Source: CAD feature listing. Evaluate the final solid. Frame: model axes, mm. Face numbers are marked on the shaded views. A direction names the side the tool comes from. Coordinates: 2 decimals unless noted, no trailing zeros. Order: outer loops, then holes, each group sorted by start corner. A loop starts at its lowest first (then second) coordinate and runs counter-clockwise, first axis right, second up.
Item 1: Section C-C on x = 0. Return the cut outline in (y, z) (3 decimals), then the cut area to 3 significant figures.
Item 2: Ray query, line 1 (X direction, y = 42, z = -19.05); line 2 (X direction, y = 58.5, z = -17); line 3 (Z direction, x = 3, y = 45). Return the intervals inside material, ascending.
Item 3: Section D-D on z = 3. Return the cut outline in (x, y), then the cut area to 3 significant figures.
Item 4: Mould query, pull axis Y, two halves, no side actions, for the marked faces 5, 6, 7 and 8. Classes: released by +Y, released by -Y, zero draft, split by the parting line, or undercut.
Item 5: Contact query for flat-ended pins moving along their axis: P1, Ø4, axis at x = 35, z = -46.5, coming from the -Y side; P2, Ø10, axis at x = -77.5, y = 7.5, coming from the +Z side; P3, Ø2, axis at y = 50.5, z = -28, coming from the -X side. Output: stop coordinate, or through.
Item 6: Reachability of the marked faces 1, 2, 3 and 4 from +Z, -Z, +X, -X, +Y, -Y: full face, straight path, thin tool, end or side. Return the list, or none.
Item 7: Section B-B on y = 55.5. State how many separate pieces and enclosed holes the cut face has, then the cut area to 3 significant figures.
Item 8: Section A-A on z = 19.05. Return the cut outline in (x, y) (3 decimals), then the cut area to 3 significant figures.
from build123d import *

# Parameters (mm, degrees)
BOSS_EXTRUDE1_DEPTH   = 38.1
BOSS_EXTRUDE1_2_DEPTH = 38.1
BOSS_EXTRUDE2_DEPTH   = 50.8
SKETCH2_R             = 6.35
CUT_EXTRUDE2_DEPTH    = 28.575
SKETCH3_W             = 38.1
SKETCH3_H             = 101.6
CUT_EXTRUDE3_DEPTH    = 12.7


with BuildPart() as part:
    # Sketch1 → Boss-Extrude1 (new, symmetric)
    with BuildSketch(Plane.XY):
        with BuildLine():
            Line((50.8, 0), (114.3, 0))
            Line((114.3, 0), (114.3, 38.1))
            Line((114.3, 38.1), (88.9, 38.1))
            Line((88.9, 38.1), (88.9, 63.5))
            Line((88.9, 63.5), (76.2, 63.5))
            ThreePointArc((76.2, 63.5), (66.900640303, 41.049359697), (44.45, 31.75))
            Line((44.45, 31.75), (19.05, 31.75))
            Line((19.05, 31.75), (19.05, 12.7))
            Line((19.05, 12.7), (63.5, 12.7))
            Line((63.5, 12.7), (50.8, 0))
        make_face()
    extrude(amount=BOSS_EXTRUDE1_DEPTH, both=True)



with BuildPart() as body_2:
    # Sketch1 → Boss-Extrude1 2 (new, symmetric)
    with BuildSketch(Plane.XY):
        with BuildLine():
            Line((-63.5, 12.7), (-19.05, 12.7))
            Line((-19.05, 12.7), (-19.05, 31.75))
            Line((-19.05, 31.75), (-44.45, 31.75))
            ThreePointArc((-44.45, 31.75), (-66.900640303, 41.049359697), (-76.2, 63.5))
            Line((-76.2, 63.5), (-88.9, 63.5))
            Line((-88.9, 63.5), (-88.9, 38.1))
            Line((-88.9, 38.1), (-114.3, 38.1))
            Line((-114.3, 38.1), (-114.3, 0))
            Line((-114.3, 0), (-50.8, 0))
            Line((-50.8, 0), (-63.5, 12.7))
        make_face()
    extrude(amount=BOSS_EXTRUDE1_2_DEPTH, both=True)


with BuildPart() as part_1:
    add(part.part)

    add(body_2.part)  # Boss-Extrude2 merges body 2
    # Sketch1<3> → Boss-Extrude2 (add, symmetric)
    with BuildSketch(Plane.XY):
        with BuildLine():
            Line((19.05, 0), (19.05, 12.7))
            Line((19.05, 12.7), (19.05, 31.75))
            Line((19.05, 31.75), (44.45, 31.75))
            ThreePointArc((44.45, 31.75), (66.900640303, 41.049359697), (76.2, 63.5))
            Line((76.2, 63.5), (63.5, 63.5))
            ThreePointArc((63.5, 63.5), (44.45, 44.45), (25.4, 63.5))
            Line((25.4, 63.5), (0, 63.5))
            Line((0, 63.5), (0, 0))
            Line((0, 0), (19.05, 0))
        make_face()
        with BuildLine():
            Line((-19.05, 0), (0, 0))
            Line((0, 0), (0, 63.5))
            Line((0, 63.5), (-25.4, 63.5))
            ThreePointArc((-25.4, 63.5), (-44.45, 44.45), (-63.5, 63.5))
            Line((-63.5, 63.5), (-76.2, 63.5))
            ThreePointArc((-76.2, 63.5), (-66.900640303, 41.049359697), (-44.45, 31.75))
            Line((-44.45, 31.75), (-19.05, 31.75))
            Line((-19.05, 31.75), (-19.05, 12.7))
            Line((-19.05, 12.7), (-19.05, 0))
        make_face()
    extrude(amount=BOSS_EXTRUDE2_DEPTH, both=True)

    # Sketch2 → Cut-Extrude2 (cut)
    with BuildSketch(Plane(origin=(0, 63.5, 0), x_dir=(1, 0, 0), z_dir=(0, 1, 0))):
        with Locations(Location((-76.2, 19.05, 0), (0, 0, 270))):
            Circle(SKETCH2_R)
        with Locations(Location((0, 38.1, 0), (0, 0, 270))):
            Circle(SKETCH2_R)
        with Locations(Location((76.2, 19.05, 0), (0, 0, 90))):
            Circle(SKETCH2_R)
        with Locations(Location((76.2, -19.05, 0), (0, 0, 270))):
            Circle(SKETCH2_R)
        with Locations(Location((0, -38.1, 0), (0, 0, 90))):
            Circle(SKETCH2_R)
        with Locations(Location((-76.2, -19.05, 0), (0, 0, 90))):
            Circle(SKETCH2_R)
    extrude(amount=-CUT_EXTRUDE2_DEPTH, mode=Mode.SUBTRACT)

    # Sketch3 → Cut-Extrude3 (cut)
    with BuildSketch(Plane.XZ):
        Rectangle(SKETCH3_W, SKETCH3_H)
    extrude(amount=-CUT_EXTRUDE3_DEPTH, mode=Mode.SUBTRACT)


solid = part_1.part
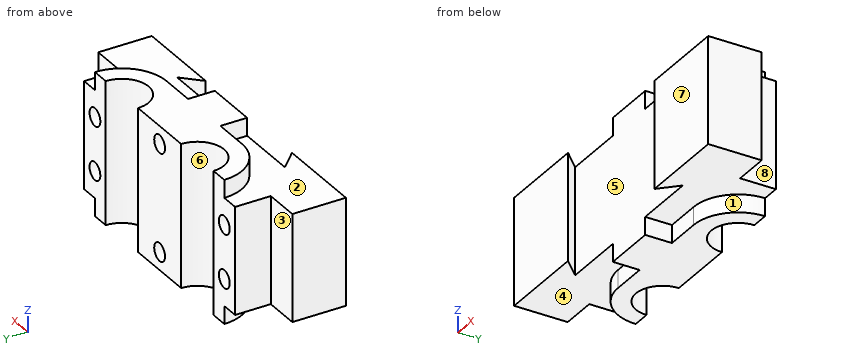
Answer list:
1. outline: (12.7, -50.8) - (63.5, -50.8) - (63.5, -44.45) - (34.925, -44.45) - (34.925, -31.75) - (63.5, -31.75) - (63.5, 31.75) - (34.925, 31.75) - (34.925, 44.45) - (63.5, 44.45) - (63.5, 50.8) - (12.7, 50.8) - close
1. area: 4,440 mm2
2. line 1: x = -88.9 to -82.55, -69.85 to 69.85, 82.55 to 88.9
2. line 2: x = -88.9 to -82.21, -70.19 to -62.83, -26.07 to 26.07, 62.83 to 70.19, 82.21 to 88.9
2. line 3: z = -50.8 to -43.7, -32.5 to 32.5, 43.7 to 50.8
3. outline: (-114.3, 0) - (-50.8, 0) - (-63.5, 12.7) - (63.5, 12.7) - (50.8, 0) - (114.3, 0) - (114.3, 38.1) - (88.9, 38.1) - (88.9, 63.5) - (63.5, 63.5) arc R19.05 cw to (25.4, 63.5) - (-25.4, 63.5) arc R19.05 cw to (-63.5, 63.5) - (-88.9, 63.5) - (-88.9, 38.1) - (-114.3, 38.1) - close
3. area: 10,600 mm2
4. face 5: undercut
4. face 6: released by +Y
4. face 7: released by -Y
4. face 8: zero draft
5. P1: stops at y = 31.75
5. P2: stops at z = 38.1
5. P3: stops at x = -88.9
6. face 1: -Z, +X, -Y
6. face 2: +Z, -X, -Y
6. face 3: +Z, -Z, -X, +Y
6. face 4: -Z, -X, -Y
7. separate pieces: 3
7. enclosed holes: 6
7. area: 9,580 mm2
8. outline: (-114.3, 0) - (-50.8, 0) - (-63.5, 12.7) - (63.5, 12.7) - (50.8, 0) - (114.3, 0) - (114.3, 38.1) - (88.9, 38.1) - (88.9, 63.5) - (82.55, 63.5) - (82.55, 34.925) - (69.85, 34.925) - (69.85, 63.5) - (63.5, 63.5) arc R19.05 cw to (25.4, 63.5) - (-25.4, 63.5) arc R19.05 cw to (-63.5, 63.5) - (-69.85, 63.5) - (-69.85, 34.925) - (-82.55, 34.925) - (-82.55, 63.5) - (-88.9, 63.5) - (-88.9, 38.1) - (-114.3, 38.1) - close
8. area: 9,910 mm2
